Source: CAD feature listing. Evaluate the final solid. Frame: model axes, mm. A direction names the side the tool comes from. Coordinates: 2 decimals unless noted, no trailing zeros. Write each loop counter-clockwise with the first axis right and the second up, starting at its lowest first coordinate (ties: lowest second). Pieces come first, ordered by that corner, then holes. Notation, with made-up numbers: M 60,49 L 77,49 A32 cw 77,82 Z; hole C 81,2 d1. An arc over 180 degrees is marked long. Answer as CSV lines item,"result". Start each with the question number.
1. Reachability of faces 1 (the face through (22, -16.9, 0)), 2 (the face through (20, -15, 0)), 3 (the face through (21, -5, -20)) from +Z, -Z, +X, -X, +Y, -Y: full face, straight path, thin tool, end or side. Return the list, or none.
2. Section A-A on y = -19.5. Return the cut outline in (x, z), plus the area to 3 significant figures.
3. Contact query for flat-ended pins moving along their axis: pin 1 Ø1 at (x, y) = (19, -11) entering from -Z; pin 2 Ø8 at (x, y) = (17, -29.5) entering from -Z; pin 3 Ø10.5 at (x, z) = (0, 0) entering from -Y; pin 4 Ø6 at (x, z) = (2.5, 12) entering from +Y. Output: stop coordinate, or through.
4. Line query: probe 1 along Y at (x, z) = (22, -2.5); probe 2 along Y at (x, z) = (11, -16); probe 3 along Y at (x, z) = (1, -6). Output: solid intervals per line, ascending. Write a range as [from, to].
5. Section D-D on z = -15. Return the cut outline in (x, y), plus the area to 3 significant figures.
6. Mould query, pull axis Y, two halves, no side actions, for faces 4 (the face through (22, -19.4, 12.6)), 5 (the face through (22, -34, 15)), 6 (the face through (11, 4, -9)). Classes: pulls with the +Y half, pulls with the -Y half, needs draft (parallel to the pull), parting line crosses it, or undercut.
7. Section C-C on z = 0. Count the separate pieces of the cut face and the enclosed holes in it, plus the area to 3 significant figures.
```python
from build123d import *

# Parameters (mm, degrees)
SKETCH1_W               = 40
SKETCH1_H               = 40
SKETCH1_R               = 4
BOSS_EXTRUDE1_DEPTH     = 4
SKETCH2_R               = 9
SKETCH2_R_2             = 4
BOSS_EXTRUDE2_DEPTH     = 5
SKETCH3_W               = 40
SKETCH3_H               = 43
BOSS_EXTRUDE3_DEPTH     = 4
CUT_EXTRUDE1_DEPTH      = 60.338014797
CUT_EXTRUDE1_DEPTH_BACK = 60.338014797
CHAMFER2_SIZE           = 5
CHAMFER3_SIZE           = 10


with BuildPart() as part:
    # Sketch1 → Boss-Extrude1 (new body)
    with BuildSketch(Plane(origin=(0, 0, 0), x_dir=(1, 0, 0), z_dir=(0, 1, 0))):
        Rectangle(SKETCH1_W, SKETCH1_H)
        with Locations(Location((0, 0, 0), (0, 0, 270))):
            Circle(SKETCH1_R, mode=Mode.SUBTRACT)
    extrude(amount=BOSS_EXTRUDE1_DEPTH)

    # Sketch2 → Boss-Extrude2 (add)
    with BuildSketch(Plane(origin=(0, 4, 0), x_dir=(1, 0, 0), z_dir=(0, 1, 0))):
        with Locations(Location((0, 0, 0), (0, 0, 270))):
            Circle(SKETCH2_R)
        with Locations(Location((0, 0, 0), (0, 0, 270))):
            Circle(SKETCH2_R_2, mode=Mode.SUBTRACT)
    extrude(amount=BOSS_EXTRUDE2_DEPTH)

    # Sketch3 → Boss-Extrude3 (add)
    with BuildSketch(Plane(origin=(20, 0, 0), x_dir=(0, 0, -1), z_dir=(1, 0, 0))):
        with Locations((0, -17.5)):
            Rectangle(SKETCH3_W, SKETCH3_H)
    extrude(amount=BOSS_EXTRUDE3_DEPTH)

    # Sketch4 → Cut-Extrude1 (cut, two sides: drawn at the far end of the back side and taken through both)
    with BuildSketch(Plane.ZY.offset(-20).offset(-CUT_EXTRUDE1_DEPTH_BACK)):
        with BuildLine():
            Line((-10, -16.9), (10, -16.9))
            ThreePointArc((10, -16.9), (12.6, -19.5), (10, -22.1))
            Line((10, -22.1), (-10, -22.1))
            ThreePointArc((-10, -22.1), (-12.6, -19.5), (-10, -16.9))
        make_face()
    extrude(amount=CUT_EXTRUDE1_DEPTH + CUT_EXTRUDE1_DEPTH_BACK, mode=Mode.SUBTRACT)

    # Chamfer2
    chamfer2_edges = [part.edges().sort_by_distance(p)[0] for p in [
        (0, 4, -9),
    ]]
    chamfer(chamfer2_edges, length=CHAMFER2_SIZE - 0.0001)  # a hair under: the kernel refuses the full size

    # Chamfer3
    chamfer3_edges = [part.edges().sort_by_distance(p)[0] for p in [
        (22, -39, 20),
        (22, -39, -20),
        (-20, 2, 20),
        (-20, 2, -20),
    ]]
    chamfer(chamfer3_edges, length=CHAMFER3_SIZE)


solid = part.part
```
Values:
1,face 1,"+X, -X"
1,face 2,"+Z, -Z, -X, -Y"
1,face 3,"-Z, +X, -X, +Y, -Y"
2,outline,"M 20,-20 L 24,-20 L 24,-12.6 L 20,-12.6 Z; M 20,12.6 L 24,12.6 L 24,20 L 20,20 Z"
2,area,"59.2 mm²"
3,pin 1,"through"
3,pin 2,"z = -20"
3,pin 3,"y = 0"
3,pin 4,"y = 8.74"
4,probe 1,"[-39, -22.1], [-16.9, 4]"
4,probe 2,"[0, 4]"
4,probe 3,"[0, 9]"
5,outline,"M -15,0 L 20,0 L 20,-34 L 24,-34 L 24,4 L -15,4 Z"
5,area,"292 mm²"
6,face 4,"undercut"
6,face 5,"pulls with the -Y half"
6,face 6,"pulls with the +Y half"
7,separate pieces,"3"
7,enclosed holes,"0"
7,area,"354 mm²"
